For this review, use the dimensioned drawing (mm, ordinates from the lowest corner) and the shaded views. A direction names the side the tool comes from. Round coordinates to 2 decimals unless told otherwise and drop trailing zeros. Order: outer loops, then holes, each group sorted by start corner. A loop starts at its lowest first (then second) coordinate and runs counter-clockwise, first axis right, second up. Notation, with made-up numbers: M 16,43.25 L 54,43.25 A9 cw 54,48.25 Z; hole C 39,1 d10. An arc over 180 degrees is marked long. Use a Markdown table: item, result. Add a question column.
1. Consider section D-D on z = 30.5. State the section outline as (x, y) points.
2. For the marked faces 5, 6 and 7, list the 3-axis set-ups (+Z, -Z, +X, -X, +Y, -Y) from which the entire face can be reached by the end or side of a thin tool; tool diameter is ignored.
3. To check wall thickness, follow probe 1 along Y at (x, z) = (35, 2); probe 2 along Z at (x, y) = (14.5, 14.25); probe 3 along Z at (x, y) = (46.5, 14.25). State the ranges of each line that lie inside material, in increasing order.
4. Consider section B-B on x = 35. State the section outline as (y, z) points, then the cut area to 3 significant figures.
5. Insertion check: P1, Ø1.7, axis at x = 5.6, z = 30.5, coming from the -Y side; P2, Ø20.5, axis at x = 29, z = 23.5, coming from the +Y side; P3, Ø5.5, axis at x = 15.5, y = 15.5, coming from the -Z side. Each pin has a flat end and moves straight along its axis. Give the tip position at first contact, or say it passes through.
6. The part is to be moulded in two halves that separate along X. For the marked faces 1, 2, 3 and 4, say which applies: +X half, -X half, draft (parallel to the pull), parting line (faces both ways), or undercut.
7. Consider section A-A on z = 23.5. State the section outline as (x, y) points, then the cut area to 3 significant figures.
8. Consider section C-C on y = 15. State the section outline as (x, z) points.
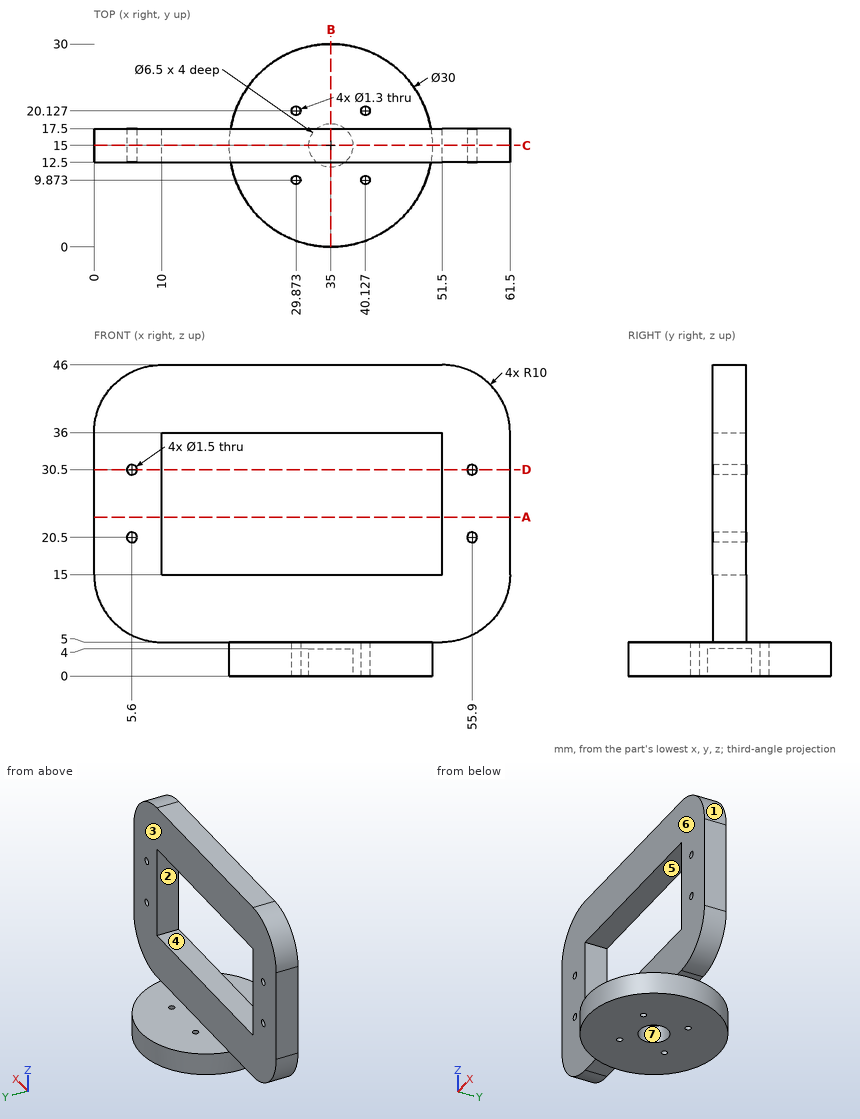
Answer block:
| question | item | result |
|---|---|---|
| 1 | outline | M 0,12.5 L 4.85,12.5 L 4.85,17.5 L 0,17.5 Z; M 6.35,12.5 L 10,12.5 L 10,17.5 L 6.35,17.5 Z; M 51.5,12.5 L 55.15,12.5 L 55.15,17.5 L 51.5,17.5 Z; M 56.65,12.5 L 61.5,12.5 L 61.5,17.5 L 56.65,17.5 Z |
| 2 | face 5 | +Y, -Y |
| 2 | face 6 | +Z, +X, -X, -Y |
| 2 | face 7 | -Z |
| 3 | probe 1 | 0 to 11.75, 18.25 to 30 |
| 3 | probe 2 | 5 to 15, 36 to 46 |
| 3 | probe 3 | 0 to 15, 36 to 46 |
| 4 | outline | M 0,0 L 11.75,0 L 11.75,4 L 18.25,4 L 18.25,0 L 30,0 L 30,5 L 17.5,5 L 17.5,15 L 12.5,15 L 12.5,5 L 0,5 Z; M 12.5,36 L 17.5,36 L 17.5,46 L 12.5,46 Z |
| 4 | area | 224 mm^2 |
| 5 | P1 | y = 12.5 |
| 5 | P2 | y = 17.5 |
| 5 | P3 | z = 5 |
| 6 | face 1 | +X half |
| 6 | face 2 | undercut |
| 6 | face 3 | draft |
| 6 | face 4 | undercut |
| 7 | outline | M 0,12.5 L 10,12.5 L 10,17.5 L 0,17.5 Z; M 51.5,12.5 L 61.5,12.5 L 61.5,17.5 L 51.5,17.5 Z |
| 7 | area | 100 mm^2 |
| 8 | outline | M 0,15 A10 ccw 10,5 L 20,5 L 20,0 L 31.75,0 L 31.75,4 L 38.25,4 L 38.25,0 L 50,0 L 50,5 L 51.5,5 A10 ccw 61.5,15 L 61.5,36 A10 ccw 51.5,46 L 10,46 A10 ccw 0,36 Z; hole C 5.6,20.5 d1.5; hole C 5.6,30.5 d1.5; hole M 10,15 L 51.5,15 L 51.5,36 L 10,36 Z; hole C 55.9,20.5 d1.5; hole C 55.9,30.5 d1.5 |
